from build123d import *

# Parameters (mm, degrees)
SKETCH1_R               = 12.7
BASE_VOLUME_DEPTH       = 6.35
SKETCH2_OUTSIDE_W       = 35.02
SKETCH2_OUTSIDE_H       = 35.02
SKETCH2_OUTSIDE_R       = 7.9375
ENCAVURE_DEPTH          = 4.7625
TROU_SHAFT_D_DEPTH      = 20.05
TROU_SHAFT_D_DEPTH_BACK = 20.05


with BuildPart() as part:
    # Sketch1 → base_volume (new, symmetric)
    with BuildSketch(Plane.XY):
        Circle(SKETCH1_R)
    extrude(amount=BASE_VOLUME_DEPTH, both=True)

    # Sketch2 outside → encavure (cut, symmetric)
    with BuildSketch(Plane.XY):
        Rectangle(SKETCH2_OUTSIDE_W, SKETCH2_OUTSIDE_H)
        Circle(SKETCH2_OUTSIDE_R, mode=Mode.SUBTRACT)
    extrude(amount=ENCAVURE_DEPTH, both=True, mode=Mode.SUBTRACT)

    # Sketch3 → trou_shaft_D (cut, two sides: drawn at the far end of the back side and taken through both)
    with BuildSketch(Plane.XY.offset(-TROU_SHAFT_D_DEPTH_BACK)):
        with BuildLine():
            Line((-1.9, 2.574878638), (1.9, 2.574878638))
            ThreePointArc((1.9, 2.574878638), (0, -3.2), (-1.9, 2.574878638))
        make_face()
    extrude(amount=TROU_SHAFT_D_DEPTH + TROU_SHAFT_D_DEPTH_BACK, mode=Mode.SUBTRACT)


solid = part.part
Read the model definition and answer for the solid it produces. Units are mm, in the model's axes. A direction names the side the tool comes from. Coordinates: 2 decimals unless noted, no trailing zeros. Loops run counter-clockwise (first coordinate to the right, second up) from the corner with the lowest first, then second, coordinate; pieces in that order, holes last.
Q1. The mould has two halves that part along Y. Classify faces 1 (the face through (-2.75, -12.4, 5.57)), 2 (the face through (0, 2.575, 0)), 3 (the face through (-0.2, -8.3, -4.762)): +Y half, -Y half, draft (parallel to the pull), parting line (faces both ways), or undercut.
Q2. The part is cut by section A-A on x = 0. Write down the section's boundary in (y, z), and give its area (3 significant figures).
Q3. Consider probe 1 along Y at (x, z) = (0, -1); probe 2 along Z at (x, y) = (9.5, 7.25). Determine where each line is inside the solid, lowest interval first.
Q4. The part is cut by section C-C on x = -4.75. Write down the section's boundary in (y, z).
Q5. The part is cut by section B-B on y = -6.5. Write down the section's boundary in (x, z), and give its area (3 significant figures).
Q6. Each of these flat-tipped pins is pushed along its axis until it touches: pin 1 Ø4 at (x, y) = (0, 0) entering from +Z; pin 2 Ø4 at (y, z) = (-5, -2.5) entering from -X; pin 3 Ø2 at (x, z) = (-3.5, -1.5) entering from -Y; pin 4 Ø6 at (y, z) = (6, -3) entering from +X. Where does it stop, or does it pass through?
Q7. The part is cut by section D-D on z = -2.25. Write down the section's boundary in (x, y) (1 decimal), and give its area (3 significant figures).
Q8. Which of the six approach directions +Z, -Z, +X, -X, +Y, -Y give full straight-line access (tool end or side, diameter ignored) to faces 4 (the face through (-2.75, -12.4, -5.55)), 5 (the face through (-1.72, -7.75, -0.07))?
Results below:
1. face 1: parting line
1. face 2: undercut
1. face 3: draft
2. outline: (-12.7, -6.35) - (-3.2, -6.35) - (-3.2, 6.35) - (-12.7, 6.35) - (-12.7, 4.76) - (-7.94, 4.76) - (-7.94, -4.76) - (-12.7, -4.76) - close; (2.57, -6.35) - (12.7, -6.35) - (12.7, -4.76) - (7.94, -4.76) - (7.94, 4.76) - (12.7, 4.76) - (12.7, 6.35) - (2.57, 6.35) - close
2. area: 159 mm2
3. probe 1: y = -7.94 to -3.2, 2.57 to 7.94
3. probe 2: z = -6.35 to -4.76, 4.76 to 6.35
4. outline: (-11.78, -6.35) - (11.78, -6.35) - (11.78, -4.76) - (6.36, -4.76) - (6.36, 4.76) - (11.78, 4.76) - (11.78, 6.35) - (-11.78, 6.35) - (-11.78, 4.76) - (-6.36, 4.76) - (-6.36, -4.76) - (-11.78, -4.76) - close
5. outline: (-10.91, -6.35) - (10.91, -6.35) - (10.91, -4.76) - (4.56, -4.76) - (4.56, 4.76) - (10.91, 4.76) - (10.91, 6.35) - (-10.91, 6.35) - (-10.91, 4.76) - (-4.56, 4.76) - (-4.56, -4.76) - (-10.91, -4.76) - close
5. area: 156 mm2
6. pin 1: passes through
6. pin 2: stops at x = -7.35
6. pin 3: stops at y = -7.53
6. pin 4: stops at x = 12.19
7. outline: circle Ø15.9 at (0, 0); hole (-1.9, 2.6) arc R3.2 ccw (long way) to (1.9, 2.6) - close
7. area: 167 mm2
8. face 4: +Z, -Z
8. face 5: none
